Model file for the job. Use its own axes, mm. A direction names the side the tool comes from. Coordinates: 2 decimals unless noted, no trailing zeros. Order: outer loops, then holes, each group sorted by start corner. A loop starts at its lowest first (then second) coordinate and runs counter-clockwise, first axis right, second up.
from build123d import *

# Parameters (mm, degrees)
SKETCH1_W           = 0.64
SKETCH1_H           = 0.64
BOSS_EXTRUDE1_DEPTH = 10


with BuildPart() as part:
    # Sketch1 → Boss-Extrude1 (new body)
    with BuildSketch(Plane.XY):
        Polygon((0, 4.92), (10.28, 4.92), (10.28, 0), (8.96, 0), (8.96, 1.9), (1.32, 1.9), (1.32, 0), (0, 0), align=None)
        with Locations((6.471040223, 3.602802159)):
            Rectangle(SKETCH1_W, SKETCH1_H, mode=Mode.SUBTRACT)
        with Locations((1.278959777, 3.602802159)):
            Rectangle(SKETCH1_W, SKETCH1_H, mode=Mode.SUBTRACT)
        with Locations((3.808959777, 3.602802159)):
            Rectangle(SKETCH1_W, SKETCH1_H, mode=Mode.SUBTRACT)
        with Locations((9.001040223, 3.602802159)):
            Rectangle(SKETCH1_W, SKETCH1_H, mode=Mode.SUBTRACT)
    extrude(amount=-BOSS_EXTRUDE1_DEPTH)


solid = part.part
Q1. Cut at B-B, the plane z = -5.75. List the corners of the cut face in (x, y), plus the area to 3 significant figures.
Established:
outline: (0, 0) - (1.32, 0) - (1.32, 1.9) - (8.96, 1.9) - (8.96, 0) - (10.28, 0) - (10.28, 4.92) - (0, 4.92) - close; hole (0.96, 3.28) - (1.6, 3.28) - (1.6, 3.92) - (0.96, 3.92) - close; hole (3.49, 3.28) - (4.13, 3.28) - (4.13, 3.92) - (3.49, 3.92) - close; hole (6.15, 3.28) - (6.79, 3.28) - (6.79, 3.92) - (6.15, 3.92) - close; hole (8.68, 3.28) - (9.32, 3.28) - (9.32, 3.92) - (8.68, 3.92) - close
area: 34.4 mm2
Q2. Which spindle directions (+Z, -Z, +X, -X, +Y, -Y) get a long thin tool onto all of the face, cutting with end or side? Do faces 1 (the face through (5, 1.9, -5)), 2 (the face through (5, 3, 0)). Say none if no direction does.
Established:
face 1: +Z, -Z, -Y
face 2: +Z, +X, -X, +Y, -Y
Q3. Cut at A-A, the plane y = 3.65. List the corners of the cut face in (x, z).
Established:
outline: (0, -10) - (0.96, -10) - (0.96, 0) - (0, 0) - close; (1.6, -10) - (3.49, -10) - (3.49, 0) - (1.6, 0) - close; (4.13, -10) - (6.15, -10) - (6.15, 0) - (4.13, 0) - close; (6.79, -10) - (8.68, -10) - (8.68, 0) - (6.79, 0) - close; (9.32, -10) - (10.28, -10) - (10.28, 0) - (9.32, 0) - close
Q4. Mould opens along X. For faces 3 (the face through (1, 0, -5)), 4 (the face through (10.28, 2, -5)), 5 (the face through (0, 2, -5)), 6 (the face through (1.32, 1, -5)) say: pulls with the +X half, pulls with the -X half, needs draft (parallel to the pull), parting line crosses it, or undercut.
Established:
face 3: needs draft
face 4: pulls with the +X half
face 5: pulls with the -X half
face 6: undercut
Q5. Cut at D-D, the plane x = 4.5. List the corners of the cut face in (y, z), plus the area to 3 significant figures.
Established:
outline: (1.9, -10) - (4.92, -10) - (4.92, 0) - (1.9, 0) - close
area: 30.2 mm2
Q6. Drop flat-ended pins along their axis: P1, Ø0.7, axis at x = 9, z = -3.5, coming from the -Y side; P2, Ø4, axis at x = 6, z = -6, coming from the -Y side. Give the stop position or say it passes through.
Established:
P1: stops at y = 0
P2: stops at y = 1.9
Q7. Probe line 1 (X direction, y = 3.45, z = -1.5); line 2 (X direction, y = 1, z = -4.75); line 3 (Y direction, x = 1, z = -4.75). List the from-to ranges inside material, lowest first.
Established:
line 1: x = 0 to 0.96, 1.6 to 3.49, 4.13 to 6.15, 6.79 to 8.68, 9.32 to 10.28
line 2: x = 0 to 1.32, 8.96 to 10.28
line 3: y = 0 to 3.28, 3.92 to 4.92
Q8. Cut at C-C, the plane y = 1.45. List the corners of the cut face in (x, z).
Established:
outline: (0, -10) - (1.32, -10) - (1.32, 0) - (0, 0) - close; (8.96, -10) - (10.28, -10) - (10.28, 0) - (8.96, 0) - close
